Here's how the part is built. I have some questions about the finished solid (model axes, mm). Face numbers are marked on the shaded views. A direction names the side the tool comes from. Give positions to 0.01 mm unless a question says otherwise; leave off trailing zeros. Order: outer loops, then holes, each group sorted by start corner. A loop starts at its lowest first (then second) coordinate and runs counter-clockwise, first axis right, second up. Notation, with made-up numbers: M 35.5,-24 L 39.5,-24 A6 ccw 39.5,-17 Z; hole C 10,67.5 d9. An arc over 180 degrees is marked long. Use one line per item in the form item = value.
Autodesk Inventor part; units mm, degrees
ref_plane "YZ Plane" through (0, 0, 0) normal (1, 0, 0) x (0, 1, 0)
ref_plane "XZ Plane" through (0, 0, 0) normal (0, 1, 0) x (-1, 0, 0)
ref_plane "XY Plane" through (0, 0, 0) normal (0, 0, 1) x (1, 0, 0)
sketch "Sketch1" plane through (0, 0, 0) normal (0, 1, 0) x (-1, 0, 0)
  line L0 (0, 0) -> (21.717, 0)
  line L1 (0, 0) -> (0, -12.7)
  line L2 (21.717, 0) -> (24.765, 0)
  line L3 (24.765, 0) -> (24.765, -3.81)
  line L4 (24.765, -3.81) -> (21.717, 0)
  line L5 (24.765, 0) -> (25.4, 0)
  line L6 (25.4, 0) -> (25.4, -3.81)
  line L7 (25.4, -3.81) -> (24.765, -3.81)
  line L8 (24.765, -3.81) -> (24.765, 0)
  line L9 (25.4, 0) -> (21.59, 0)
  line L10 (21.59, 0) -> (21.59, 1.905)
  line L11 (21.59, 1.905) -> (25.4, 1.905)
  line L12 (25.4, 1.905) -> (25.4, 0)
  dimension "d0" = 21.717
  dimension "d1" = 12.7
  dimension "d2" = 3.048
  dimension "d3" = 3.81
  dimension "d4" = 0.635
  dimension "d6" = 1.905
revolve "Revolution1" add sketch "Sketch1" angle 360 about axis through (0, 0, 0) along (0, 0, -1)
sketch "Sketch3" plane through (0, 0, -3.81) normal (0, 0, -1) x (-1, 0, 0)
  circle A0 centre (0, 0) radius 25.4
  circle A1 centre (0, 0) radius 34.925
  line L0 (0, 0) -> (0, 34.925)
  line L1 (0, 0) -> (-24.6957, 24.6957)
  line L2 (0, 0) -> (34.925, 0) construction
  circle A2 centre (0, 0) radius 25.4
  line L3 (0, 0) -> (-30.2459, -17.4625)
  line L4 (0, 0) -> (34.925, 0) construction
  line L5 (0, 0) -> (-9.0393, -33.735)
  line L6 (0, 0) -> (34.925, 0) construction
  line L7 (0, 0) -> (30.2459, -17.4625)
  line L8 (0, 0) -> (34.925, 0) construction
  line L9 (0, 0) -> (33.735, 9.0393)
  line L10 (0, 0) -> (34.925, 0) construction
  arc A3 (0, 25.4) -> (-17.9605, 17.9605) centre (0, 0) ccw
  arc A4 (-21.997, -12.7) -> (-6.574, -24.5345) centre (0, 0) ccw
  arc A5 (21.997, -12.7) -> (24.5345, 6.574) centre (0, 0) ccw
  dimension "d7" = 69.85
  dimension "d8" = 135
  dimension "d9" = 150
  dimension "d10" = 105
  dimension "d11" = 30
  dimension "d12" = 15
extrude "Extrusion1" add sketch "Sketch3" against normal blind 2.54 contours A0 L9 A1 L7 | A0 L1 A1 L0 | L5 A1 L3 A0
properties part number "FanMount" material "PC/ABS Plastic"
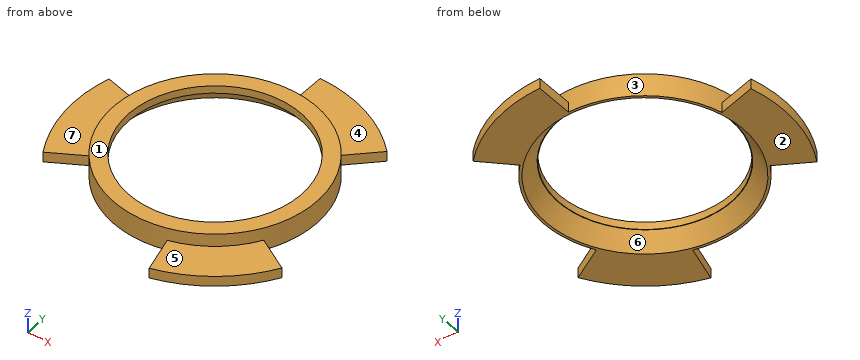
Q1. I want a section at C-C on y = -27. Write out the boundary of the cut face in (x, z).
Found:
outline = M 7.23,-3.81 L 22.15,-3.81 L 22.15,-1.27 L 7.23,-1.27 Z
Q2. I need wall thicknesses on L1, parallel to Y at x = 0, z = 0.5; L2, parallel to X at y = -17, z = -2.2; L3, parallel to Z at x = 9.5, y = -28. Which ranges of each line are inside material? Lowest first, please.
Found:
L1 = -25.4 to -21.59, 21.59 to 25.4
L2 = -30.51 to -29.44, -18.87 to -16.19, 16.19 to 29.44
L3 = -3.81 to -1.27
Q3. I want a section at D-D on y = 29.5. Write out the boundary of the cut face in (x, z), then the cut area to 3 significant figures.
Found:
outline = M 0,-3.81 L 18.7,-3.81 L 18.7,-1.27 L 0,-1.27 Z
area = 47.5 mm²
Q4. On a 3-axis mill with a long thin cutter (end or side, diameter ignored), from which of +Z, -Z, +X, -X, +Y, -Y can I reach the whole of each face in a straight line? I mean the marked faces 1, 2, 3, 4 and 5. Say none if no direction works.
Found:
face_1 = +Z, +X, -X, +Y, -Y
face_2 = -Z, +X, -X, +Y, -Y
face_3 = +Z
face_4 = +Z, +X, +Y
face_5 = +Z, +X, -Y
Q5. I'm going to push flat-ended pins straight in: pin 1 Ø1.3 at (y, z) = (31, -2) entering from -X; pin 2 Ø2 at (y, z) = (3, -1.5) entering from +X; pin 3 Ø3 at (y, z) = (13, -2.5) entering from +X. Where does each tip first touch, or does it pass through?
Found:
pin_1 = 0
pin_2 = 25.32
pin_3 = 22.65
Q6. Thinking about a two-plate mould opening in Y: for the marked faces 6 and 7, which applies, +Y half, -Y half, draft (parallel to the pull), parting line (faces both ways), or undercut?
Found:
face_6 = undercut
face_7 = draft
Q7. I want a section at A-A on y = 0. Write out the boundary of the cut face in (x, z) (3 decimals), then the cut area to 3 significant figures.
Found:
outline = M -34.925,-3.81 L -24.765,-3.81 L -21.717,0 L -21.59,0 L -21.59,1.905 L -25.4,1.905 L -25.4,-1.27 L -34.925,-1.27 Z; M 21.59,0 L 21.717,0 L 24.765,-3.81 L 25.4,-3.81 L 25.4,1.905 L 21.59,1.905 Z
area = 55.2 mm²
